```python
from build123d import *

# Parameters (mm, degrees)
SKETCH008_W  = 18
SKETCH008_H  = 5
PAD008_DEPTH = 4
SKETCH010_W  = 9.9
SKETCH010_H  = 1.99
PAD009_DEPTH = 4
SKETCH011_W  = 12
SKETCH011_H  = 1.8
PAD010_DEPTH = 4


with BuildPart() as part:
    # Sketch008 → Pad008 (new body)
    with BuildSketch(Plane(origin=(0, -10.4875, 0), x_dir=(-1, 0, 0), z_dir=(0, 1, 0))):
        with Locations((0, -1.5)):
            Rectangle(SKETCH008_W, SKETCH008_H)
    extrude(amount=-PAD008_DEPTH)

    # Sketch010 → Pad009 (new body)
    with BuildSketch(Plane(origin=(0, -10.4875, 1), x_dir=(1, 0, 0), z_dir=(0, 0, 1))):
        with Locations((0, -2.995)):
            Rectangle(SKETCH010_W, SKETCH010_H)
    extrude(amount=PAD009_DEPTH)

    # Sketch011 → Pad010 (new body)
    with BuildSketch(Plane(origin=(0, -14.4875, 0), x_dir=(-1, 0, 0), z_dir=(0, -1, 0))):
        with Locations((0, 3.1)):
            Rectangle(SKETCH011_W, SKETCH011_H)
    extrude(amount=PAD010_DEPTH)


solid = part.part
```
Here's how the part is built. I have some questions about the finished solid (model axes, mm). A direction names the side the tool comes from. Coordinates: 2 decimals unless noted, no trailing zeros. Order: outer loops, then holes, each group sorted by start corner. A loop starts at its lowest first (then second) coordinate and runs counter-clockwise, first axis right, second up.
1) Imagine slicing it at B-B on y = -13.5. List the corners of the cut face in (x, z) for me, and give its area (3 significant figures).
2) Which directions (+Z, -Z, +X, -X, +Y, -Y) give clear straight access to the entire face, cutting with the end or side of a thin tool? Please do faces 1 (the face through (0, -14.478, 3)), 2 (the face through (4.95, -13, 3)), 3 (the face through (0, -12.488, 3)), 4 (the face through (6, -16, -3)).
3) Imagine slicing it at A-A on z = -3.5. List the corners of the cut face in (x, y) for me, and give its area (3 significant figures).
4) Imagine slicing it at D-D on z = 3.25. List the corners of the cut face in (x, y) for me, and give its area (3 significant figures).
5) Will these pins go through, and if not, where does the flat tip stop? pin 1 (2 mm diameter, centred on x = -3, y = -17.5, fed in from +Z); pin 2 (0.6 mm diameter, centred on y = -13.5, z = 3, fed in from -X); pin 3 (1.5 mm diameter, centred on y = -17.5, z = -1, fed in from -X); pin 4 (2 mm diameter, centred on x = 0.5, z = 3, fed in from -Y).
6) I need wall thicknesses on line 1 (Z direction, x = -2.5, y = -15.5); line 2 (Y direction, x = -1.75, z = 2.25); line 3 (Y direction, x = 5.75, z = 0). Which ranges of each line are inside material? Lowest first, please.
Response values:
1. outline: (-9, -4) - (9, -4) - (9, 1) - (4.95, 1) - (4.95, 5) - (-4.95, 5) - (-4.95, 1) - (-9, 1) - close
1. area: 130 mm2
2. face 1: +Z, +X, -X, -Y
2. face 2: +Z, +X, +Y, -Y
2. face 3: +Z, +X, -X, +Y
2. face 4: +Z, -Z, +X, -Y
3. outline: (-9, -14.49) - (-6, -14.49) - (-6, -18.49) - (6, -18.49) - (6, -14.49) - (9, -14.49) - (9, -10.49) - (-9, -10.49) - close
3. area: 120 mm2
4. outline: (-4.95, -14.48) - (4.95, -14.48) - (4.95, -12.49) - (-4.95, -12.49) - close
4. area: 19.7 mm2
5. pin 1: stops at z = -2.2
5. pin 2: stops at x = -4.95
5. pin 3: passes through
5. pin 4: stops at y = -14.48
6. line 1: z = -4 to -2.2
6. line 2: y = -14.48 to -12.49
6. line 3: y = -14.49 to -10.49
